Part model, mm, in its own coordinate system. Face numbers are marked on the shaded views. A direction names the side the tool comes from. Round coordinates to 2 decimals unless told otherwise and drop trailing zeros. Order: outer loops, then holes, each group sorted by start corner. A loop starts at its lowest first (then second) coordinate and runs counter-clockwise, first axis right, second up. Notation, with made-up numbers: (-22, 71) - (36, 71) arc R10 ccw to (36, 84) - close; hole circle Ø5 at (29, -25.75). An arc over 180 degrees is marked (long way). Return JSON: item names as keys, results as strings. Group by question number.
Item 1: Saw through at C-C on y = 0.5. List the corners of the cut face in (x, z).
Item 2: Drop flat-ended pins along their axis: pin 1 (0.6 mm diameter, centred on x = 6, y = 2, fed in from +Z); pin 2 (1.5 mm diameter, centred on x = -3, y = 1, fed in from +Z); pin 3 (0.6 mm diameter, centred on x = -5.5, y = 1, fed in from +Z). Give the stop position or say it passes through.
Item 3: Probe probe 1 along Y at (x, z) = (-1, 4.5); probe 2 along X at (y, z) = (3.7, 0); probe 3 along X at (y, z) = (1.15, 1.25). List the from-to ranges inside material, lowest first.
Item 4: Saw through at D-D on y = 2.55. List the corners of the cut face in (x, z), and give its area (3 significant figures).
Item 5: Tool access for the marked faces 1, 2 and 3: list every direction of +Z, -Z, +X, -X, +Y, -Y with a clear straight run to the whole face (end or side of a thin tool).
Item 6: Two-plate mould, pull along X, no slides. Class the marked faces 4, 5 and 6: released by +X, released by -X, zero draft, split by the parting line, or undercut.
Item 7: Saw through at B-B on x = 0.5. List the corners of the cut face in (y, z).
Item 8: Saw through at A-A on y = 1.8. List the corners of the cut face in (x, z).
```python
from build123d import *

# Parameters (mm, degrees)
SKETCH1_R           = 1.5
BOSS_EXTRUDE1_DEPTH = 1
BOSS_EXTRUDE2_DEPTH = 1
CIRPATTERN1_COUNT   = 4
SKETCH4_R           = 2
SKETCH4_R_2         = 1.5
BOSS_EXTRUDE3_DEPTH = 4


with BuildPart() as part:
    # Sketch1 → Boss-Extrude1 (new body)
    with BuildSketch(Plane(origin=(0, 0, 0), x_dir=(1, 0, 0), z_dir=(0, 1, 0))):
        with BuildLine():
            Line((-5.2, 3.9), (-5.2, 0))
            Line((-5.2, 0), (-6.5, 0))
            Line((-6.5, 0), (-6.5, -1))
            Line((-6.5, -1), (-6.422616289, -1))
            ThreePointArc((-6.422616289, -1), (-5.572172087, -3.346774303), (-3.9, -5.2))
            Line((-3.9, -5.2), (0, -5.2))
            Line((0, -5.2), (0, -6.5))
            Line((0, -6.5), (1, -6.5))
            Line((1, -6.5), (1, -6.422616289))
            ThreePointArc((1, -6.422616289), (3.346774303, -5.572172087), (5.2, -3.9))
            Line((5.2, -3.9), (5.2, 0))
            Line((5.2, 0), (6.5, 0))
            Line((6.5, 0), (6.5, 1))
            Line((6.5, 1), (6.422616289, 1))
            ThreePointArc((6.422616289, 1), (5.572172087, 3.346774303), (3.9, 5.2))
            Line((3.9, 5.2), (0, 5.2))
            Line((0, 5.2), (0, 6.5))
            Line((0, 6.5), (-1, 6.5))
            Line((-1, 6.5), (-1, 6.422616289))
            ThreePointArc((-1, 6.422616289), (-3.346774303, 5.572172087), (-5.2, 3.9))
        make_face()
        with Locations(Location((0, 0, 0), (0, 0, 270))):
            Circle(SKETCH1_R, mode=Mode.SUBTRACT)
    extrude(amount=BOSS_EXTRUDE1_DEPTH)

    # Sketch3 → Boss-Extrude2 (add)
    with BuildSketch(Plane.ZY):
        Polygon((5.2, 1), (5.2, 3), (5.6, 3), (6.5, 1), align=None)
    boss_extrude2 = extrude(amount=-BOSS_EXTRUDE2_DEPTH)

    # CirPattern1: Boss-Extrude2 ×4 about axis
    cirpattern1_axis = Axis((0, 0, 0), (0, 1, 0))
    for i in range(1, CIRPATTERN1_COUNT):
        add(boss_extrude2.rotate(cirpattern1_axis, i * 360 / CIRPATTERN1_COUNT))

    # Sketch4 → Boss-Extrude3 (add)
    with BuildSketch(Plane(origin=(0, 1, 0), x_dir=(1, 0, 0), z_dir=(0, 1, 0))):
        with Locations(Location((0, 0, 0), (0, 0, 270))):
            Circle(SKETCH4_R)
        with Locations(Location((0, 0, 0), (0, 0, 270))):
            Circle(SKETCH4_R_2, mode=Mode.SUBTRACT)
    extrude(amount=BOSS_EXTRUDE3_DEPTH)


solid = part.part
```
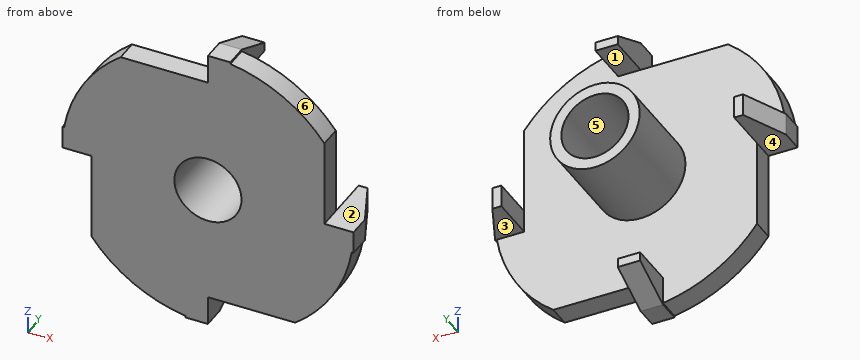
Filled in:
{
 "1": {"outline": "(-6.5, 0) - (-5.2, 0) - (-5.2, -3.9) arc R6.5 ccw to (-1, -6.42) - (-1, -6.5) - (0, -6.5) - (0, -5.2) - (3.9, -5.2) arc R6.5 ccw to (6.42, -1) - (6.5, -1) - (6.5, 0) - (5.2, 0) - (5.2, 3.9) arc R6.5 ccw to (1, 6.42) - (1, 6.5) - (0, 6.5) - (0, 5.2) - (-3.9, 5.2) arc R6.5 ccw to (-6.42, 1) - (-6.5, 1) - close; hole circle Ø3 at (0, 0)"},
 "2": {"pin 1": "stops at z = 0", "pin 2": "stops at z = 5.2", "pin 3": "stops at z = 3.9"},
 "3": {"probe 1": "y = 0 to 1", "probe 2": "x = -2 to -1.5, 1.5 to 2", "probe 3": "x = -1.56 to -0.83, 0.83 to 1.56"},
 "4": {"outline": "(-5.8, 0) - (-5.2, 0) - (-5.2, 1) - (-5.8, 1) - close; circle Ø4 at (0, 0); (-1, -5.8) - (0, -5.8) - (0, -5.2) - (-1, -5.2) - close; (0, 5.2) - (1, 5.2) - (1, 5.8) - (0, 5.8) - close; (5.2, -1) - (5.8, -1) - (5.8, 0) - (5.2, 0) - close; hole circle Ø3 at (0, 0)", "area": "7.91 mm^2"},
 "5": {"face 1": "+X, -X, +Y", "face 2": "+Z, +X, +Y, -Y", "face 3": "-Z, +X, +Y"},
 "6": {"face 4": "zero draft", "face 5": "undercut", "face 6": "released by +X"},
 "7": {"outline": "(0, -5.2) - (1, -5.2) - (1, -1.94) - (5, -1.94) - (5, -1.41) - (0, -1.41) - close; (0, 1.41) - (5, 1.41) - (5, 1.94) - (1, 1.94) - (1, 5.2) - (3, 5.2) - (3, 5.6) - (1, 6.5) - (0, 6.5) - close"},
 "8": {"outline": "(-6.14, 0) - (-5.2, 0) - (-5.2, 1) - (-6.14, 1) - close; circle Ø4 at (0, 0); (-1, -6.14) - (0, -6.14) - (0, -5.2) - (-1, -5.2) - close; (0, 5.2) - (1, 5.2) - (1, 6.14) - (0, 6.14) - close; (5.2, -1) - (6.14, -1) - (6.14, 0) - (5.2, 0) - close; hole circle Ø3 at (0, 0)"}
}
